Work out the finished part from the listing and answer in its coordinate system (mm). Face numbers are marked on the shaded views. Give positions to 0.01 mm unless a question says otherwise; leave off trailing zeros. Write each loop counter-clockwise with the first axis right and the second up, starting at its lowest first coordinate (ties: lowest second). Pieces come first, ordered by that corner, then holes. Notation, with made-up numbers: (81.5, -20) - (113.5, -20) arc R27 cw to (113.5, 0) - close; hole circle Ø1 at (50.25, -34). An arc over 180 degrees is marked (long way). Write item = value, one per line.
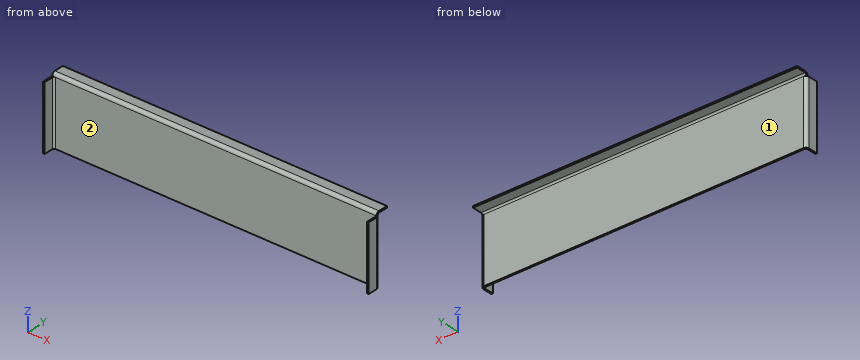
from build123d import *

# Parameters (mm, degrees)
SKETCH1_W                    = 489.688000048
SKETCH1_H                    = 101.6
BASE_FLANGE1_DEPTH           = 2.3622
EDGE_FLANGE1_STRIP_W         = 14.1688
EDGE_FLANGE1_STRIP_H         = 2.3622
EDGE_FLANGE1_STRIP_CUT_DEPTH = 489.688000048
EDGE_FLANGE1_DEPTH           = 489.688000048
EDGE_FLANGE2_STRIP_W         = 14.1688
EDGE_FLANGE2_STRIP_H         = 2.3622
EDGE_FLANGE2_STRIP_CUT_DEPTH = 96.8778
EDGE_FLANGE2_DEPTH           = 96.8778
EDGE_FLANGE3_STRIP_W         = 14.1688
EDGE_FLANGE3_STRIP_H         = 2.3622
EDGE_FLANGE3_STRIP_CUT_DEPTH = 96.8778
EDGE_FLANGE3_DEPTH           = 96.8778


# Sheet-metal steps are written as plain solids
with BuildPart() as part:
    # Sketch1 → Base-Flange1 (new body)
    with BuildSketch(Plane(origin=(0, 0, 0), x_dir=(1, 0, 0), z_dir=(0, 1, 0))):
        Rectangle(SKETCH1_W, SKETCH1_H)
    extrude(amount=-BASE_FLANGE1_DEPTH)

    # Edge-Flange1 strip (across the edge) → Edge-Flange1 strip cut (cut)
    with BuildSketch(Plane(origin=(-244.844000024, 0, 50.8), x_dir=(0, 0, -1), z_dir=(1, 0, 0))):
        with Locations((-2.3622, -1.1811)):
            Rectangle(EDGE_FLANGE1_STRIP_W, EDGE_FLANGE1_STRIP_H)
    extrude(amount=EDGE_FLANGE1_STRIP_CUT_DEPTH, mode=Mode.SUBTRACT)

    # Edge-Flange1 section (across the edge) → Edge-Flange1 (add)
    with BuildSketch(Plane(origin=(-244.844000024, 0, 50.8), x_dir=(0, 0, -1), z_dir=(1, 0, 0))):
        with BuildLine():
            Line((0, 2.36), (0, 16.6878))
            Line((0, 16.6878), (2.3622, 16.6878))
            Line((2.3622, 16.6878), (2.3622, 2.36))
            ThreePointArc((2.3622, 2.36), (3.053427996, 0.691227996), (4.7222, 0))
            Line((4.7222, 0), (4.7222, -2.3622))
            ThreePointArc((4.7222, -2.3622), (1.383100358, -0.979099642), (0, 2.36))
        make_face()
    extrude(amount=EDGE_FLANGE1_DEPTH)

    # Edge-Flange2 strip (across the edge) → Edge-Flange2 strip cut (cut)
    with BuildSketch(Plane(origin=(-244.844000024, -2.3622, 46.0778), x_dir=(1, 0, 0), z_dir=(0, 0, -1))):
        with Locations((-2.3622, -1.1811)):
            Rectangle(EDGE_FLANGE2_STRIP_W, EDGE_FLANGE2_STRIP_H)
    extrude(amount=EDGE_FLANGE2_STRIP_CUT_DEPTH, mode=Mode.SUBTRACT)

    # Edge-Flange2 section (across the edge) → Edge-Flange2 (add)
    with BuildSketch(Plane(origin=(-244.844000024, -2.3622, 46.0778), x_dir=(1, 0, 0), z_dir=(0, 0, -1))):
        with BuildLine():
            Line((0, 2.36), (0, 16.6878))
            Line((0, 16.6878), (2.3622, 16.6878))
            Line((2.3622, 16.6878), (2.3622, 2.36))
            ThreePointArc((2.3622, 2.36), (3.053427996, 0.691227996), (4.7222, 0))
            Line((4.7222, 0), (4.7222, -2.3622))
            ThreePointArc((4.7222, -2.3622), (1.383100358, -0.979099642), (0, 2.36))
        make_face()
    extrude(amount=EDGE_FLANGE2_DEPTH)

    # Edge-Flange3 strip (across the edge) → Edge-Flange3 strip cut (cut)
    with BuildSketch(Plane(origin=(244.844000024, -2.3622, -50.8), x_dir=(-1, 0, 0), z_dir=(0, 0, 1))):
        with Locations((-4.7244, -1.1811)):
            Rectangle(EDGE_FLANGE3_STRIP_W, EDGE_FLANGE3_STRIP_H)
    extrude(amount=EDGE_FLANGE3_STRIP_CUT_DEPTH, mode=Mode.SUBTRACT)

    # Edge-Flange3 section (across the edge) → Edge-Flange3 (add)
    with BuildSketch(Plane(origin=(244.844000024, -2.3622, -50.8), x_dir=(-1, 0, 0), z_dir=(0, 0, 1))):
        with BuildLine():
            Line((-2.3622, 2.36), (-2.3622, 16.6878))
            Line((-2.3622, 16.6878), (0, 16.6878))
            Line((0, 16.6878), (0, 2.36))
            ThreePointArc((0, 2.36), (0.691227996, 0.691227996), (2.36, 0))
            Line((2.36, 0), (2.36, -2.3622))
            ThreePointArc((2.36, -2.3622), (-0.979099642, -0.979099642), (-2.3622, 2.36))
        make_face()
    extrude(amount=EDGE_FLANGE3_DEPTH)


solid = part.part
1. For a pull along Y with two mould halves and no side action, classify the marked faces 1 and 2 as pulls with the +Y half, pulls with the -Y half, needs draft (parallel to the pull), parting line crosses it, or undercut.
Solution:
face_1 = pulls with the +Y half
face_2 = pulls with the -Y half
2. Straight lines are drawn through the part: line 1 (X direction, y = -11.5, z = 12); line 2 (Z direction, x = -222.5, y = 14.5); line 3 (Y direction, x = 224.5, z = 3). For each, find the intervals that lie inside material, in ascending order.
Solution:
line_1 = -244.84 to -242.48, 244.84 to 247.21
line_2 = 48.44 to 50.8
line_3 = -2.36 to 0
3. Find section B-B, the plane x = -109. Give the vertices of the cut face in (y, z), then the cut area to 3 significant figures.
Solution:
outline = (-2.36, -50.8) - (0, -50.8) - (0, 46.08) arc R2.36 cw to (2.36, 48.44) - (16.69, 48.44) - (16.69, 50.8) - (2.36, 50.8) arc R4.72 ccw to (-2.36, 46.08) - close
area = 276 mm^2
4. Find section A-A, the plane y = -14. Give the vertices of the cut face in (x, z), then the cut area to 3 significant figures.
Solution:
outline = (-244.84, -50.8) - (-242.48, -50.8) - (-242.48, 46.08) - (-244.84, 46.08) - close; (244.84, -50.8) - (247.21, -50.8) - (247.21, 46.08) - (244.84, 46.08) - close
area = 458 mm^2
5. Find section D-D, the plane y = 11.5. Give the vertices of the cut face in (x, z), then the cut area to 3 significant figures.
Solution:
outline = (-244.84, 48.44) - (244.84, 48.44) - (244.84, 50.8) - (-244.84, 50.8) - close
area = 1,160 mm^2
6. Find section C-C, the plane z = -22.5. Give the vertices of the cut face in (x, y), then the cut area to 3 significant figures.
Solution:
outline = (-244.84, -19.05) - (-242.48, -19.05) - (-242.48, -4.72) arc R2.36 cw to (-240.12, -2.36) - (242.48, -2.36) arc R2.36 cw to (244.84, -4.72) - (244.84, -19.05) - (247.21, -19.05) - (247.21, -4.72) arc R4.72 ccw to (242.48, 0) - (-240.12, 0) arc R4.72 ccw to (-244.84, -4.72) - close
area = 1,230 mm^2
7. Given pin 1 (1.5 mm diameter, centred on x = -108, y = 13, fed in from -Z); pin 2 (12 mm diameter, centred on x = -174, z = -27.5, fed in from -Y); pin 3 (4 mm diameter, centred on x = -73.5, z = 38.5, fed in from +Y), each flat-ended and moving along its own axis, determine where each tip first touches the part or whether it passes through.
Solution:
pin_1 = 48.44
pin_2 = -2.36
pin_3 = 0
